Here's how the part is built. I have some questions about the finished solid (model axes, mm). A direction names the side the tool comes from. Coordinates: 2 decimals unless noted, no trailing zeros. Order: outer loops, then holes, each group sorted by start corner. A loop starts at its lowest first (then second) coordinate and runs counter-clockwise, first axis right, second up. Notation, with made-up numbers: M 79,-15 L 93,-15 A16 ccw 93,-1 Z; hole C -8.75,58 d5. An arc over 180 degrees is marked long. Answer as CSV lines item,"result". Start each with the question number.
```python
from build123d import *

# Parameters (mm, degrees)
CUT_EXTRUDE_1_DEPTH = 4
FILLET_1_R          = 1
SKETCH_3_R          = 1
CUT_EXTRUDE_2_DEPTH = 4
SKETCH_4_R          = 1
CUT_EXTRUDE_3_DEPTH = 4


with BuildPart() as part:
    # 草图1 → 旋转1 (revolve)
    with BuildSketch(Plane.XY, mode=Mode.PRIVATE) as revolve_1_sk:
        Polygon((2, 0), (2, 2), (3, 2), (3, 4), (3.5, 4), (3.5, 12.5), (10, 12.5), (10, 7.5), (8, 0.918629754), (2.2, 0), align=None)
    revolve(revolve_1_sk.sketch.rotate(Axis((0, 0.286130796, 0), (0, -1, 0)), 180), axis=Axis((0, 0.286130796, 0), (0, -1, 0)))

    # 草图2 → 切除-拉伸1 (cut)
    with BuildSketch(Plane(origin=(0, 12.5, 0), x_dir=(1, 0, 0), z_dir=(0, 1, 0))):
        with BuildLine():
            Line((-7.416198487, 3), (-4, 3))
            ThreePointArc((-4, 3), (0, 5), (4, 3))
            Line((4, 3), (7.416198487, 3))
            ThreePointArc((7.416198487, 3), (8, 0), (7.416198487, -3))
            Line((7.416198487, -3), (4, -3))
            ThreePointArc((4, -3), (0, -5), (-4, -3))
            Line((-4, -3), (-7.416198487, -3))
            ThreePointArc((-7.416198487, -3), (-8, 0), (-7.416198487, 3))
        make_face()
    extrude(amount=-CUT_EXTRUDE_1_DEPTH, mode=Mode.SUBTRACT)

    # 圆角1
    fillet_1_edges = [part.edges().sort_by_distance(p)[0] for p in [
        (-7.416198487, 10.5, 3),
        (-7.416198487, 10.5, -3),
        (-4, 10.5, -3),
        (4, 10.5, -3),
        (7.416198487, 10.5, -3),
        (7.416198487, 10.5, 3),
        (4, 10.5, 3),
        (-4, 10.5, 3),
    ]]
    fillet(fillet_1_edges, radius=FILLET_1_R)

    # 草图3 → 切除-拉伸2 (cut)
    with BuildSketch(Plane(origin=(0, 8.5, 0), x_dir=(1, 0, 0), z_dir=(0, 1, 0))):
        with Locations(Location((5.5, 0, 0), (0, 0, 180))):
            Circle(SKETCH_3_R)
        with Locations((-5.5, 0)):
            Circle(SKETCH_3_R)
    extrude(amount=-CUT_EXTRUDE_2_DEPTH, mode=Mode.SUBTRACT)

    # 草图4 → 切除-拉伸3 (cut)
    with BuildSketch(Plane(origin=(0, 12.5, 0), x_dir=(1, 0, 0), z_dir=(0, 1, 0))):
        with Locations(Location((-4.5, 6, 0), (0, 0, 180))):
            Circle(SKETCH_4_R)
        with Locations(Location((4.5, 6, 0), (0, 0, 180))):
            Circle(SKETCH_4_R)
        with Locations(Location((-4.5, -6, 0), (0, 0, 180))):
            Circle(SKETCH_4_R)
        with Locations(Location((4.5, -6, 0), (0, 0, 180))):
            Circle(SKETCH_4_R)
    extrude(amount=-CUT_EXTRUDE_3_DEPTH, mode=Mode.SUBTRACT)


solid = part.part
```
1) Suppose I cut it at D-D on y = 6.75. Please give me the cut outline in (x, z), plus the area to 3 significant figures.
2) Suppose I cut it at C-C on y = 10. Please give me the cut outline in (x, z), plus the area to 3 significant figures.
3) Which directions (+Z, -Z, +X, -X, +Y, -Y) give clear straight access to the entire face, cutting with the end or side of a thin tool? Please do faces 4 (the face through (10, 10, 0)), 5 (the face through (7.299, 10.472, 2.807)).
4) I need wall thicknesses on line 1 (Z direction, x = -5, y = 11.25); line 2 (Z direction, x = 3.75, y = 10); line 3 (X direction, y = 11.75, z = -2.75). Which ranges of each line are inside material? Lowest first, please. Write a range as [from, to].
5) If we mould it in two halves opening along Z, with no side actions, what happens to faces 1 (the face through (-7.935, 1.969, -2.499)), 2 (the face through (-8, 11, 0)), 3 (the face through (2, 12.5, -5))? For each: released by +Z, released by -Z, zero draft, split by the parting line, or undercut.
6) Will these pins go through, and if not, where does the flat tip stop? pin 1 Ø3.5 at (x, z) = (0, 0) entering from -Y; pin 2 Ø3 at (x, y) = (-6, 4.5) entering from -Z; pin 3 Ø2 at (x, z) = (-3, -4.5) entering from -Y; pin 4 Ø6.5 at (x, z) = (0, 0) entering from -Y.
7) Suppose I cut it at B-B on x = 0. Please give me the cut outline in (y, z), plus the area to 3 significant figures.
Output:
1,outline,"C 0,0 d19.54; hole C -5.5,0 d2; hole C 0,0 d7; hole C 5.5,0 d2"
1,area,"255 mm²"
2,outline,"C 0,0 d20; hole M -7.67,-2.29 A1 ccw -6.71,-3 L -4.47,-3 A1 cw -3.73,-3.33 A5 ccw 3.73,-3.33 A1 cw 4.47,-3 L 6.71,-3 A1 ccw 7.67,-2.29 A8 ccw 7.67,2.29 A1 ccw 6.71,3 L 4.47,3 A1 cw 3.73,3.33 A5 ccw -3.73,3.33 A1 cw -4.47,3 L -6.71,3 A1 ccw -7.67,2.29 A8 ccw Z; hole C -4.5,-6 d2; hole C -4.5,6 d2; hole C 4.5,-6 d2; hole C 4.5,6 d2"
2,area,"186 mm²"
3,face 4,"+Y, -Y"
3,face 5,"+Y"
4,line 1,"[-8.66, -6.87], [-5.13, -3], [3, 5.13], [6.87, 8.66]"
4,line 2,"[-9.27, -6.66], [-5.34, -3.31], [3.31, 5.34], [6.66, 9.27]"
4,line 3,"[-9.61, -7.37], [7.37, 9.61]"
5,face 1,"split by the parting line"
5,face 2,"undercut"
5,face 3,"zero draft"
6,pin 1,"through"
6,pin 2,"z = -8.04"
6,pin 3,"y = 0.35"
6,pin 4,"y = 0"
7,outline,"M 0,-2.2 L 0.92,-8 L 7.5,-10 L 12.5,-10 L 12.5,-5 L 8.5,-5 L 8.5,-3.5 L 4,-3.5 L 4,-3 L 2,-3 L 2,-2 L 0,-2 Z; M 0,2 L 2,2 L 2,3 L 4,3 L 4,3.5 L 8.5,3.5 L 8.5,5 L 12.5,5 L 12.5,10 L 7.5,10 L 0.92,8 L 0,2.2 Z"
7,area,"136 mm²"
